Autodesk Inventor part; units mm, degrees
ref_plane "YZ Plane" through (0, 0, 0) normal (1, 0, 0) x (0, 1, 0)
ref_plane "XZ Plane" through (0, 0, 0) normal (0, 1, 0) x (-1, 0, 0)
ref_plane "XY Plane" through (0, 0, 0) normal (0, 0, 1) x (1, 0, 0)
sketch "Sketch68" plane through (0, 0, 0) normal (1, 0, 0) x (0, 1, 0)
  line L0 (1, 4.6737) -> (23, 4.6737) construction
  line L1 (7.0021, -2.9903) -> (-7.0029, -0.0135)
  line L2 (7.2385, 26.8729) -> (5.7713, 27.1847)
  line L3 (2.4565, 4.3755) -> (1, 4.6737)
  line L4 (5.7713, 27.1847) -> (1, 4.6737)
  line L5 (7.2385, 26.8729) -> (2.4565, 4.3755)
  point P0 (0, 0)
  point P1 (2.225, 5.1772)
sketch "Sketch184" plane through (0, 0, 0) normal (1, 0, 0) x (0, 1, 0)
  arc A0 (-3.5, -3.0972) -> (0, -1.6204) centre (-4.281, 3.6397) ccw
  arc A1 (0, -1.6204) -> (2.2822, 2) centre (-4.3557, 3.6547) ccw
  arc A2 (2.2822, 2) -> (2.459, 4.3851) centre (-8.8285, 4.0231) ccw
  arc A3 (2.459, 4.3851) -> (2.3883, 6) centre (-72.7121, 1.9029) ccw
  line L0 (-3.5, -3.0972) -> (-3.5, -3.6807)
  arc A4 (2.3883, 6) -> (-3.5, -3.0972) centre (8.6947, -4.5362) ccw
  point P0 (0, 0)
sketch "Sketch213" plane through (0, 0, 0) normal (1, 0, 0) x (0, 1, 0)
  line L0 (13.3414, -11.8728) -> (-10.8201, 5)
  line L1 (46.9769, 13.1952) -> (16.4024, 18.5466)
  line L2 (-14, -25) -> (0.7357, -50.4491)
  line L3 (0.7357, -50.4491) -> (1.9473, -49.7476)
  line L4 (1.9473, -49.7476) -> (-11.7207, -26.1425)
  line L5 (-11.7207, -26.1425) -> (-10, -24)
  line L6 (-10, -24) -> (-10.853, -23.4043)
  line L7 (-10.853, -23.4043) -> (-11.992, -25.0353)
  line L8 (-11.992, -25.0353) -> (-13.0313, -25.7169)
  line L9 (-13.0313, -25.7169) -> (-11.992, -25.0353)
  line L10 (-13.0313, -25.7169) -> (-12.7653, -23.856)
  line L11 (-12.7653, -23.856) -> (-14, -25)
  line L12 (46.5114, 10.5356) -> (18.0034, 15.5254)
  line L13 (18.0034, 15.5254) -> (16.7759, 13.7195)
  line L14 (16.7759, 13.7195) -> (15.6891, 14.4784)
  line L15 (-11.992, -25.0353) -> (16.9748, 16.4444)
  line L16 (15.6891, 14.4784) -> (17.062, 16.4444)
  line L17 (17.062, 16.4444) -> (17.3561, 17.7094)
  line L18 (17.3561, 17.7094) -> (16.3637, 17.6698)
  line L19 (16.3637, 17.6698) -> (16.4024, 18.5466)
  line L20 (46.9769, 13.1952) -> (46.5114, 10.5356)
  point P0 (0, 0)
  point P1 (3.3399, -2.2736)
  point P2 (-1.2043, -8.7808)
  dimension "d600" = 1.4
  dimension "d601" = 2.7
  dimension "d603" = 1.265
revolve "Revolution5" add sketch "Sketch213" angle 180 mid plane about axis through (0, 13.3414, -11.8728) along (0, -0.8199, 0.5725) contours L20 L12 L13 L14 L16 L17 L18 L19 L1
sketch "Sketch214" plane through (25.3467, 2.5499, -4.3367) normal (0, -0.5725, -0.8199) x (-1, 0, 0)
  line L0 (-13.0367, 24.9829) -> (-11.8218, 25.5494)
  line L1 (-12.0166, 27.5278) -> (-14.4637, 26.3867)
  line L2 (-13.0367, 24.9829) -> (-9.6557, 17.7324)
  line L3 (-11.8218, 25.5494) -> (-8.4409, 18.2989)
  line L4 (-8.4409, 18.2989) -> (-9.6557, 17.7324)
  line L5 (-14.4637, 26.3867) -> (-1.3459, -1.7444)
  line L6 (69, 30) -> (69, 11.3718) construction
  line L7 (62.5521, 25.5326) -> (59.1711, 18.2822)
  line L8 (63.7303, 24.9832) -> (62.5521, 25.5326)
  line L9 (63.7303, 24.9832) -> (60.3493, 17.7328)
  line L10 (59.1711, 18.2822) -> (60.3493, 17.7328)
  line L11 (65.1571, 26.3867) -> (62.7101, 27.5278)
  line L12 (62.7101, 27.5278) -> (50.4789, 1.298)
  line L13 (52.0393, -1.7444) -> (65.1571, 26.3867)
  point P0 (25.3467, -4.5735)
  dimension "d606" = 0
  dimension "d612" = 1.875
  dimension "d613" = 8
  dimension "d614" = 0.7
  dimension "d615" = 0.7
extrude "Extrusion162" cut sketch "Sketch214" against normal blind 3
properties part number "A1_V1_M2_dropArm_WOK_meso_tall_VIS_lft"
Source: CAD feature listing. Evaluate the final solid. Frame: model axes, mm. A direction names the side the tool comes from. Round coordinates to 2 decimals unless told otherwise and drop trailing zeros. Answer as a JSON object with one key per item and string values. Group by question number.
Q1. Mould query, pull axis Y, two halves, no side actions, for faces 6 (the flat face through (-31.51, 12.06, -10.98)), 7 (the conical face through (0.825, 46.535, 10.695)), 8 (the flat face through (-34.41, 18.16, -13.44)). Classes: pulls with the +Y half, pulls with the -Y half, needs draft (parallel to the pull), parting line crosses it, or undercut.
Q2. Contact query for flat-ended pins moving along their axis: P1, Ø1, axis at x = 29, y = 27, coming from the -Z side; P2, Ø5, axis at y = 6, z = -2.5, coming from the -X side; P3, Ø12, axis at y = 16.5, z = 1, coming from the +X side. Output: stop coordinate, or through.
Q3. Access query for faces 1 (the cylindrical face through (0.5, 16.22, 14.1)), 2 (the conical face through (-0.701, 28.502, 16.422)), 3 (the conical face through (-0.508, 15.772, 14.597)), 4 (the flat face through (37.78, 24.11, -17.59)), 5 (the conical face through (0.513, 16.986, 14.028)). Directions: +Z, -Z, +X, -X, +Y, -Y. A direction counts if a zero-diameter tool reaches every point of the face in a straight line with its end or side. Return the directions, or none.
Q4. Ray query, line 1 (X direction, y = 6.5, z = -2.5); line 2 (X direction, y = 28, z = -3); line 3 (Z direction, x = -15.5, y = 37.5). Return the intervals inside material, ascending. Write a range as from..to.
Completed:
{
 "1": {"face 6": "pulls with the -Y half", "face 7": "pulls with the +Y half", "face 8": "undercut"},
 "2": {"P1": "z = -2.42", "P2": "x = -29.33", "P3": "x = 32.52"},
 "3": {"face 1": "-Z, -Y", "face 2": "+Z", "face 3": "-Y", "face 4": "none", "face 5": "-Z"},
 "4": {"line 1": "-28.28..-25.27, 25.27..28.28", "line 2": "-33.38..-30.06, 30.06..33.38", "line 3": "8.72..11.68"}
}
